Read the model definition and answer for the solid it produces. Units are mm, in the model's axes. A direction names the side the tool comes from. Coordinates: 2 decimals unless noted, no trailing zeros. Order: outer loops, then holes, each group sorted by start corner. A loop starts at its lowest first (then second) coordinate and runs counter-clockwise, first axis right, second up. Notation, with made-up numbers: M 26,28 L 70,28 A26 cw 70,65 Z; hole C -4,8 d1. An arc over 180 degrees is marked long. Use a Markdown table: item, result. Add a question column.
1) Find section C-C on y = 15. Write down the section's boundary in (x, z).
2) Each of these flat-tipped pins is pushed along its axis until it touches: pin 1 Ø1 at (x, z) = (57, 18.5) entering from -Y; pin 2 Ø0.9 at (x, z) = (1, 23) entering from +Y. Where does it stop, or does it pass through?
3) Find the intervals of material crossed by probe 1 along Z at (x, y) = (94.5, 15.75); probe 2 along X at (y, z) = (12.75, 8.5); probe 3 along Y at (x, z) = (87, 28.5), in increasing order. Write a range as [from, to].
4) Find section D-D on z = 33. Write down the section's boundary in (x, y).
5) For faces 5 (the face through (116.177, 15, 24)), 6 (the face through (58, 15, 48.26)), determine the directions among +Z, -Z, +X, -X, +Y, -Y from which every point of the face is accessible in a straight line to the end or side of a thin tool.
6) Find section A-A on z = 21. Write down the section's boundary in (x, y).
7) The mould has two halves that part along X. Classify faces 1 (the face through (118.023, 14, 24)), 2 (the face through (0, 11, 24)), 3 (the face through (58, 15, 0)), 4 (the face through (60, 24.13, 24)): released by +X, released by -X, zero draft, split by the parting line, or undercut.
8) Find section B-B on x = 34. Write down the section's boundary in (y, z).
from build123d import *

# Parameters (mm, degrees)
SKETCH2_W           = 118.023469291
SKETCH2_H           = 19.05
BOSS_EXTRUDE1_DEPTH = 48.26
SKETCH24_W          = 114.3
SKETCH24_H          = 43.18
CUT_EXTRUDE2_DEPTH  = 17.78
SKETCH25_W          = 12.7
SKETCH25_H          = 6.35
CUT_EXTRUDE3_DEPTH  = 6.604
FILLET1_R           = 2.54


with BuildPart() as part:
    # Sketch2 → Boss-Extrude1 (new body)
    with BuildSketch(Plane.XY):
        with Locations((59.011734646, 15.875)):
            Rectangle(SKETCH2_W, SKETCH2_H)
    extrude(amount=BOSS_EXTRUDE1_DEPTH)

    # Sketch24 → Cut-Extrude2 (cut)
    with BuildSketch(Plane(origin=(0, 6.35, 0), x_dir=(-1, 0, 0), z_dir=(0, -1, 0))):
        with Locations((-59.026642295, -23.975075688)):
            Rectangle(SKETCH24_W, SKETCH24_H)
    extrude(amount=-CUT_EXTRUDE2_DEPTH, mode=Mode.SUBTRACT)

    # Sketch25 → Cut-Extrude3 (cut)
    with BuildSketch(Plane.ZY):
        with Locations((24.105050581, 15.863147592)):
            Rectangle(SKETCH25_W, SKETCH25_H)
    extrude(amount=-CUT_EXTRUDE3_DEPTH, mode=Mode.SUBTRACT)

    # Fillet1
    fillet1_edges = [part.edges().sort_by_distance(p)[0] for p in [
        (59.011734646, 25.4, 48.26),
        (59.011734646, 25.4, 0),
        (0, 25.4, 24.13),
        (118.023469291, 25.4, 24.13),
    ]]
    fillet(fillet1_edges, radius=FILLET1_R)


solid = part.part
Check result:
| question | item | result |
|---|---|---|
| 1 | outline | M 0,0 L 118.02,0 L 118.02,48.26 L 0,48.26 L 0,30.46 L 1.88,30.46 L 1.88,45.57 L 116.18,45.57 L 116.18,2.39 L 1.88,2.39 L 1.88,17.76 L 0,17.76 Z |
| 2 | pin 1 | stops at y = 24.13 |
| 2 | pin 2 | stops at y = 25.15 |
| 3 | probe 1 | z = [0, 2.39], [45.57, 48.26] |
| 3 | probe 2 | x = [0, 1.88], [116.18, 118.02] |
| 3 | probe 3 | y = [24.13, 25.4] |
| 4 | outline | M 0,6.35 L 1.88,6.35 L 1.88,24.13 L 116.18,24.13 L 116.18,6.35 L 118.02,6.35 L 118.02,22.86 A2.54 ccw 115.48,25.4 L 2.54,25.4 A2.54 ccw 0,22.86 Z |
| 5 | face 5 | -Y |
| 5 | face 6 | +Z, +X, -X, +Y, -Y |
| 6 | outline | M 0,6.35 L 1.88,6.35 L 1.88,12.69 L 0,12.69 Z; M 0,19.04 L 1.88,19.04 L 1.88,24.13 L 116.18,24.13 L 116.18,6.35 L 118.02,6.35 L 118.02,22.86 A2.54 ccw 115.48,25.4 L 2.54,25.4 A2.54 ccw 0,22.86 Z |
| 7 | face 1 | released by +X |
| 7 | face 2 | released by -X |
| 7 | face 3 | zero draft |
| 7 | face 4 | undercut |
| 8 | outline | M 6.35,0 L 22.86,0 A2.54 ccw 25.4,2.54 L 25.4,45.72 A2.54 ccw 22.86,48.26 L 6.35,48.26 L 6.35,45.57 L 24.13,45.57 L 24.13,2.39 L 6.35,2.39 Z |
